Study the drawing (mm; zero at the part's minimum x, y, z) and answer. Round coordinates to 2 decimals unless told otherwise and drop trailing zeros. Write each loop counter-clockwise with the first axis right and the second up, starting at its lowest first coordinate (ties: lowest second). Pieces come first, ordered by that corner, then holes. Notation, with made-up numbers: (55, 6.25) - (77, 6.25) arc R23 cw to (77, 20.25) - close; hole circle Ø8 at (11.5, -2). An arc over 180 degrees is marked (long way). Return JSON: item names as keys, results as strings. Group by question number.
(1) Find the intervals of material crossed by line 1 along Y through (x, z) = (2.5, 20); line 2 along X through (y, z) = (2.35, 9); line 3 along X through (y, z) = (1.9, 33), in increasing order. Write a range as [from, to].
(2) This flat-tipped pin is pushed along its axis until it touches: pin 1 (1.5 mm diameter, centred on y = 4.5, z = 8.5, fed in from -X). Where does it stop, or does it pass through?
(3) Section C-C, the plane z = 28.5 is taken. Write down the section's boundary in (x, y).
(4) Section A-A, the plane y = 2.5 is taken. Write down the section's boundary in (x, z), then the cut area to 3 significant figures.
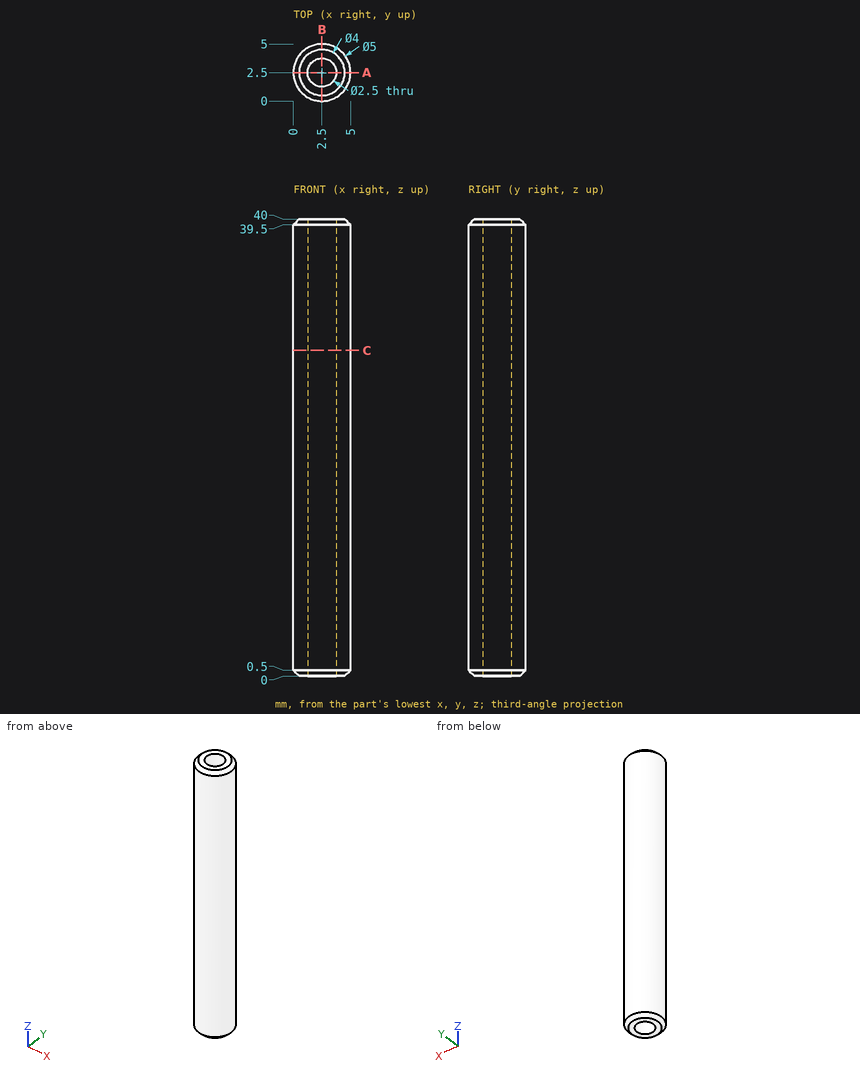
Working result:
{
 "1": {"line 1": "y = [0, 1.25], [3.75, 5]", "line 2": "x = [0, 1.26], [3.74, 5]", "line 3": "x = [0.07, 1.4], [3.6, 4.93]"},
 "2": {"pin 1": "stops at x = 0.33"},
 "3": {"outline": "circle Ø5 at (2.5, 2.5); hole circle Ø2.5 at (2.5, 2.5)"},
 "4": {"outline": "(0, 0.5) - (0.5, 0) - (1.25, 0) - (1.25, 40) - (0.5, 40) - (0, 39.5) - close; (3.75, 0) - (4.5, 0) - (5, 0.5) - (5, 39.5) - (4.5, 40) - (3.75, 40) - close", "area": "99.5 mm^2"}
}
